from build123d import *

# Parameters (mm, degrees)
ESBO_O2_R                  = 1.5
CORTE_EXTRUS_O1_DEPTH      = 127.487894678
CORTE_EXTRUS_O2_DEPTH      = 127.487894678
CORTE_EXTRUS_O2_DEPTH_BACK = 127.487894678
ESBO_O3_R                  = 4.25


with BuildPart() as part:
    # Esboço1 → Revolução1 (revolve)
    with BuildSketch(Plane(origin=(0, 0, 0), x_dir=(0, 0, -1), z_dir=(1, 0, 0)), mode=Mode.PRIVATE) as revolu_o1_sk:
        Polygon((2.5, 91.149139381), (22.25, 91.149139381), (24.25, 89.149139381), (24.25, 82.149139381), (15.5, 82.149139381), (15.5, -119.75), (13.5, -121.75), (0, -121.75), (0, -81.75), (1.5, -80.848709071), (1.5, 81.149139381), (2.5, 81.75), align=None)
    revolve(revolu_o1_sk.sketch.rotate(Axis((0, 121.75, 0), (0, -1, 0)), 180), axis=Axis((0, 121.75, 0), (0, -1, 0)))

    # Esboço2 → Corte-extrusão1 (cut, through all)
    with BuildSketch(Plane.XY):
        with Locations(Location((0, 45.799139381, 0), (0, 0, 90))):
            Circle(ESBO_O2_R)
        with Locations(Location((0, -101.500860619, 0), (0, 0, 90))):
            Circle(ESBO_O2_R)
    extrude(amount=CORTE_EXTRUS_O1_DEPTH, mode=Mode.SUBTRACT)

    # Esboço3 → Corte-extrusão2 (cut, two sides: drawn at the far end of the back side and taken through both)
    with BuildSketch(Plane.XY.offset(-CORTE_EXTRUS_O2_DEPTH_BACK)):
        with Locations((0, -112.25)):
            Circle(ESBO_O3_R)
    extrude(amount=CORTE_EXTRUS_O2_DEPTH + CORTE_EXTRUS_O2_DEPTH_BACK, mode=Mode.SUBTRACT)


solid = part.part
Geometry check sheet. Reference: the model listing, model coordinates, mm. A direction names the side the tool comes from. Give positions to 0.01 mm unless a question says otherwise; leave off trailing zeros. Write each loop counter-clockwise with the first axis right and the second up, starting at its lowest first coordinate (ties: lowest second). Pieces come first, ordered by that corner, then holes. Notation, with made-up numbers: (52, 85.25) - (62, 85.25) arc R35 ccw to (62, 119.25) - close; hole circle Ø4 at (59.25, -22.5). An arc over 180 degrees is marked (long way). Put each result on its own line as item: value.
1. Draft check along Y on faces 4 (the flat face through (16, 82.149, 0)), 5 (the cylindrical face through (2.285, -108.666, -0.219)), 6 (the conical face through (19.851, 91.024, 10.325)), 7 (the cylindrical face through (21.514, 85.6, 11.19)). Enter one of: +Y half, -Y half, draft (parallel to the pull), parting line (faces both ways), or undercut.
Ans:
face 4: -Y half
face 5: undercut
face 6: +Y half
face 7: draft
2. Sectioned sample at B-B, the plane y = -112.25. Enter the section's corners in (x, z).
Ans:
outline: (-4.25, -14.91) - (-4.25, 14.91) arc R15.5 ccw to start; (4.25, -14.91) arc R15.5 ccw to (4.25, 14.91) - close
3. Set-up check for faces 1 (the cylindrical face through (-4.656, -20.214, 14.784)), 2 (the cylindrical face through (-0.1, 86.5, -2.5)), 3 (the flat face through (5, 91.149, 0)): record each of +Z, -Z, +X, -X, +Y, -Y from which the full face is reachable in a straight line by a thin tool's end or side.
Ans:
face 1: -Y
face 2: +Y
face 3: +Z, -Z, +X, -X, +Y
4. Go/stop test with flat-tipped pins: pin 1 (4 mm diameter, centred on x = 0, y = -101.5, fed in from -Z); pin 2 (6 mm diameter, centred on x = 13, y = -29.5, fed in from -Z); pin 3 (12 mm diameter, centred on x = -9.5, y = 11.5, fed in from +Z). Record where each tip stops, or that it passes through.
Ans:
pin 1: stops at z = -15.5
pin 2: stops at z = -11.84
pin 3: stops at z = 15.1
5. Thickness scan on line 1 (X direction, y = -31, z = 0); line 2 (X direction, y = 84, z = 0); line 3 (Y direction, x = 14.5, z = -14). Record the ranges inside material, lowest first.
Ans:
line 1: x = -15.5 to -1.5, 1.5 to 15.5
line 2: x = -24.25 to -2.5, 2.5 to 24.25
line 3: y = 82.15 to 91.15
6. Sectioned sample at A-A, the plane y = -21.5. Enter the section's corners in (x, z), plus the area to 3 significant figures.
Ans:
outline: circle Ø31 at (0, 0); hole circle Ø3 at (0, 0)
area: 748 mm²
